```python
from build123d import *

# Parameters (mm, degrees)
SKETCH1_R                                      = 1.5
BOSS_EXTRUDE1_DEPTH                            = 1.3
FILLET1_R                                      = 1
BOSS_EXTRUDE3_DEPTH                            = 0.1
BOSS_EXTRUDE3_DEPTH_BACK                       = 1.4
CSK_FOR_M3_FLAT_HEAD_MACHINE_SCREW2_AT_2_COUNT = 2
CSK_FOR_M3_FLAT_HEAD_MACHINE_SCREW2_AT_2_PITCH = 11.5


with BuildPart() as part:
    # Sketch1 → Boss-Extrude1 (new body)
    with BuildSketch(Plane(origin=(0, 0, 0), x_dir=(1, 0, 0), z_dir=(0, 1, 0))):
        with BuildLine():
            Line((-11.5, 3), (11.5, 3))
            Line((11.5, 3), (11.5, -3))
            Line((11.5, -3), (9.25, -3))
            Line((9.25, -3), (9.25, -5))
            ThreePointArc((9.25, -5), (5.75, -8.5), (2.25, -5))
            Line((2.25, -5), (2.25, -3))
            Line((2.25, -3), (-2.25, -3))
            Line((-2.25, -3), (-2.25, -5))
            ThreePointArc((-2.25, -5), (-5.75, -8.5), (-9.25, -5))
            Line((-9.25, -5), (-9.25, -3))
            Line((-9.25, -3), (-11.5, -3))
            Line((-11.5, -3), (-11.5, 3))
        make_face()
        with Locations(Location((5.75, -5, 0), (0, 0, 270))):
            Circle(SKETCH1_R, mode=Mode.SUBTRACT)
        with Locations(Location((-5.75, -5, 0), (0, 0, 270))):
            Circle(SKETCH1_R, mode=Mode.SUBTRACT)
    extrude(amount=BOSS_EXTRUDE1_DEPTH)

    # Fillet1
    fillet1_edges = [part.edges().sort_by_distance(p)[0] for p in [
        (9.25, 0.65, 3),
        (2.25, 0.65, 3),
        (-2.25, 0.65, 3),
        (-9.25, 0.65, 3),
        (-11.5, 0.65, 3),
        (-11.5, 0.65, -3),
        (11.5, 0.65, -3),
        (11.5, 0.65, 3),
    ]]
    fillet(fillet1_edges, radius=FILLET1_R)

    # Sketch5 → Boss-Extrude3 (add, two sides: drawn at the far end of the back side and taken through both)
    with BuildSketch(Plane(origin=(0, 1.3, 0), x_dir=(1, 0, 0), z_dir=(0, 1, 0)).offset(-BOSS_EXTRUDE3_DEPTH_BACK)):
        Polygon((-11, -1.25), (-9, -1.25), (-9, 1.25), (-9.375, 1.25), (-9.375, 3), (-10.625, 3), (-10.625, 1.25), (-11, 1.25), align=None)
        Polygon((-7, -1.25), (-5, -1.25), (-5, 1.25), (-5.375, 1.25), (-5.375, 3), (-6.625, 3), (-6.625, 1.25), (-7, 1.25), align=None)
        Polygon((-3, -1.25), (-1, -1.25), (-1, 1.25), (-1.375, 1.25), (-1.375, 3), (-2.625, 3), (-2.625, 1.25), (-3, 1.25), align=None)
        Polygon((1, -1.25), (3, -1.25), (3, 1.25), (2.625, 1.25), (2.625, 3), (1.375, 3), (1.375, 1.25), (1, 1.25), align=None)
        Polygon((5, -1.25), (7, -1.25), (7, 1.25), (6.625, 1.25), (6.625, 3), (5.375, 3), (5.375, 1.25), (5, 1.25), align=None)
        Polygon((9, -1.25), (11, -1.25), (11, 1.25), (10.625, 1.25), (10.625, 3), (9.375, 3), (9.375, 1.25), (9, 1.25), align=None)
    extrude(amount=BOSS_EXTRUDE3_DEPTH + BOSS_EXTRUDE3_DEPTH_BACK)

    # Sketch7 → CSK for M3 Flat Head Machine Screw2 (revolve, cut)
    with BuildSketch(Plane(origin=(5.75, 0, 5), x_dir=(0, 0, -1), z_dir=(1, 0, 0))):
        Polygon((0, 0), (0, 1.4), (1.7, 1.4), (1.7, 1.45), (3.15, 0), align=None)
    csk_for_m3_flat_head_machine_screw2 = revolve(axis=Axis((5.75, -6.35, 5), (0, 1, 0)), mode=Mode.SUBTRACT)

    # CSK for M3 Flat Head Machine Screw2 at 2: CSK for M3 Flat Head Machine Screw2 ×2
    with Locations(*[(-i * CSK_FOR_M3_FLAT_HEAD_MACHINE_SCREW2_AT_2_PITCH, 0, 0) for i in range(1, CSK_FOR_M3_FLAT_HEAD_MACHINE_SCREW2_AT_2_COUNT)]):
        add(csk_for_m3_flat_head_machine_screw2, mode=Mode.SUBTRACT)


solid = part.part
```
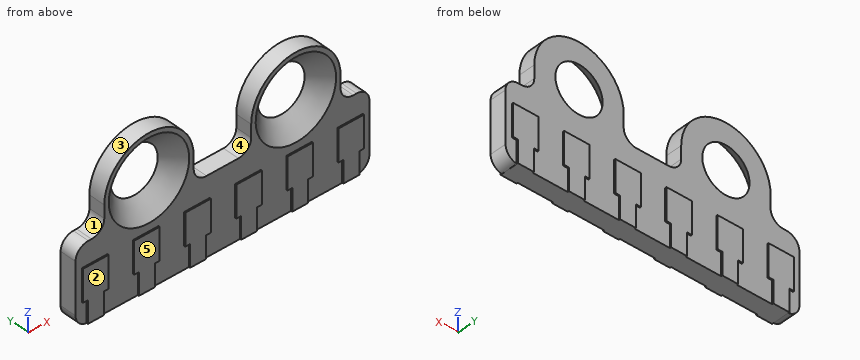
For this review, take the finished solid that the model builds, in its own axes (mm). Face numbers are marked on the shaded views. A direction names the side the tool comes from. Round coordinates to 2 decimals unless told otherwise and drop trailing zeros. Write each loop counter-clockwise with the first axis right and the second up, starting at its lowest first coordinate (ties: lowest second). Pieces come first, ordered by that corner, then holes. Notation, with made-up numbers: (12, 59.25) - (61, 59.25) arc R35 cw to (61, 91.25) - close; hole circle Ø8 at (-2.75, 84). An arc over 180 degrees is marked (long way). Write each question's results on one line, items separated by ' | '.
Item 1: Take a section at D-D on z = 6.75. Count the separate pieces of the cut face and the enclosed holes in it, then the cut area to 3 significant figures.
Calculated:
separate pieces: 4 | enclosed holes: 0 | area: 6.73 mm^2
Item 2: Take a section at A-A on y = 0.35. State the section outline as (x, z) points (3 decimals).
Calculated:
outline: (-11.5, -2) arc R1 ccw to (-10.625, -2.992) - (-10.625, -3) - (10.625, -3) - (10.625, -2.992) arc R1 ccw to (11.5, -2) - (11.5, 2) arc R1 ccw to (10.5, 3) - (10.25, 3) arc R1 cw to (9.25, 4) - (9.25, 5) arc R3.5 ccw to (2.25, 5) - (2.25, 4) arc R1 cw to (1.25, 3) - (-1.25, 3) arc R1 cw to (-2.25, 4) - (-2.25, 5) arc R3.5 ccw to (-9.25, 5) - (-9.25, 4) arc R1 cw to (-10.25, 3) - (-10.5, 3) arc R1 ccw to (-11.5, 2) - close; hole circle Ø5.6 at (-5.75, 5); hole circle Ø5.6 at (5.75, 5)
Item 3: For pin 1 (6 mm diameter, centred on x = 5.5, z = 6, fed in from -Y), flat-tipped, find the tip position at first contact; note if it passes through.
Calculated:
pin 1: stops at y = 0
Item 4: Draft analysis for pull direction X (two halves, no side actions). For the marked faces 1, 2 and 3, state which applies: pulls with the +X half, pulls with the -X half, needs draft (parallel to the pull), parting line crosses it, or undercut.
Calculated:
face 1: pulls with the -X half | face 2: needs draft | face 3: undercut
Item 5: For the marked faces 4 and 5, list the 3-axis set-ups (+Z, -Z, +X, -X, +Y, -Y) from which the entire face can be reached by the end or side of a thin tool; tool diameter is ignored.
Calculated:
face 4: +Z, +Y, -Y | face 5: +Z, -Z, +X, -X, -Y
Item 6: Take a section at B-B on x = 5.75. State the section outline as (y, z) points, then the cut area to 3 significant figures.
Calculated:
outline: (-0.1, -3) - (1.4, -3) - (1.4, 1.25) - (1.3, 1.25) - (1.3, 3.15) - (0, 1.85) - (0, 1.25) - (-0.1, 1.25) - close; (0, 8.15) - (1.3, 6.85) - (1.3, 8.5) - (0, 8.5) - close | area: 9.30 mm^2
Item 7: To check wall thickness, follow line 1 along X through (y, z) = (1.25, 4.5); line 2 along X through (y, z) = (0.8, 5); line 3 along Y through (x, z) = (8.5, -0.5). State the ranges of each line that lie inside material, in increasing order. Write a range as from..to.
Calculated:
line 1: x = -9.25..-7.58, -3.92..-2.25, 2.25..3.92, 7.58..9.25 | line 2: x = -9.25..-8.1, -3.4..-2.25, 2.25..3.4, 8.1..9.25 | line 3: y = 0..1.3
Item 8: Take a section at C-C on z = 1.5. State the section outline as (x, y) points, then the cut area to 3 significant figures.
Calculated:
outline: (-11.5, 0) - (11.5, 0) - (11.5, 1.3) - (-11.5, 1.3) - close | area: 29.9 mm^2
